The figure shows three views and two pictorial views of one solid part (mm, origin at its lowest corner). Answer the questions. Round coordinates to 2 decimals unless told otherwise and drop trailing zeros. Write each loop counter-clockwise with the first axis right and the second up, starting at its lowest first coordinate (ties: lowest second). Pieces come first, ordered by that corner, then holes.
Item 1: Find section C-C on y = 29. Give the vertices of the cut face in (x, z).
Item 2: Find section B-B on x = 62.5. Give the vertices of the cut face in (y, z), then the cut area to 3 significant figures.
Item 3: Find the intervals of material crossed by probe 1 along X at (y, z) = (49, 1.2); probe 2 along X at (y, z) = (4.5, 3.8); probe 3 along Y at (x, z) = (54, 1.4), in increasing order.
Item 4: Find section A-A on y = 42. Give the vertices of the cut face in (x, z).
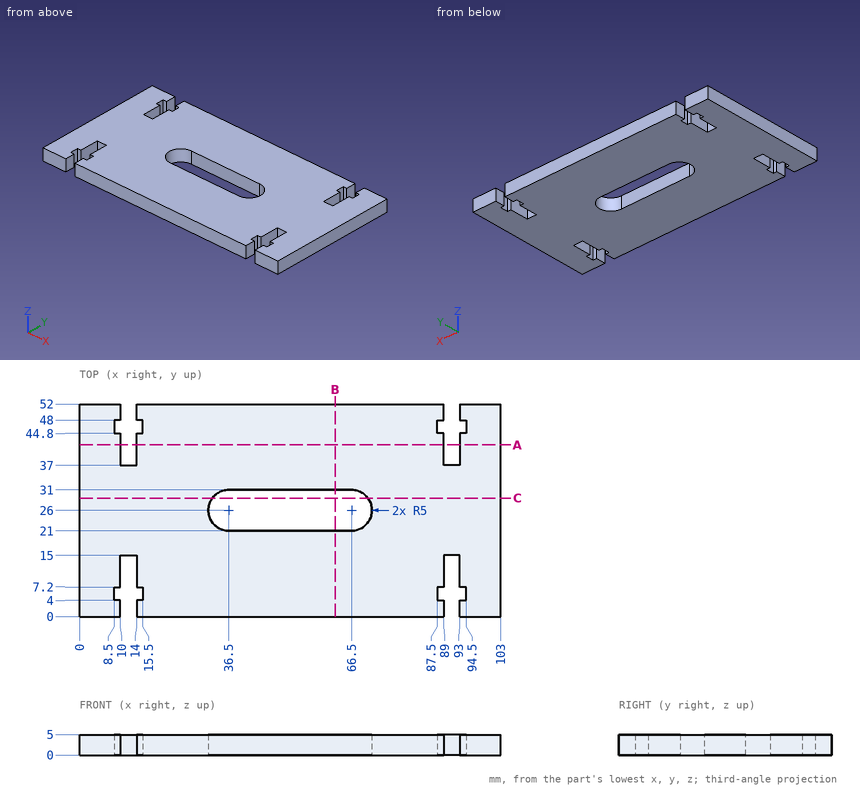
Check values:
1. outline: (0, 0) - (32.5, 0) - (32.5, 5) - (0, 5) - close; (70.5, 0) - (103, 0) - (103, 5) - (70.5, 5) - close
2. outline: (0, 0) - (21, 0) - (21, 5) - (0, 5) - close; (31, 0) - (52, 0) - (52, 5) - (31, 5) - close
2. area: 210 mm2
3. probe 1: x = 0 to 10, 14 to 89, 93 to 103
3. probe 2: x = 0 to 8.5, 15.5 to 87.5, 94.5 to 103
3. probe 3: y = 0 to 21, 31 to 52
4. outline: (0, 0) - (10, 0) - (10, 5) - (0, 5) - close; (14, 0) - (89, 0) - (89, 5) - (14, 5) - close; (93, 0) - (103, 0) - (103, 5) - (93, 5) - close
